Could you check a few things on this model? Use its own coordinates, in mm. Give positions to 0.01 mm unless a question says otherwise; leave off trailing zeros. Order: outer loops, then holes, each group sorted by start corner. A loop starts at its lowest first (then second) coordinate and runs counter-clockwise, first axis right, second up.
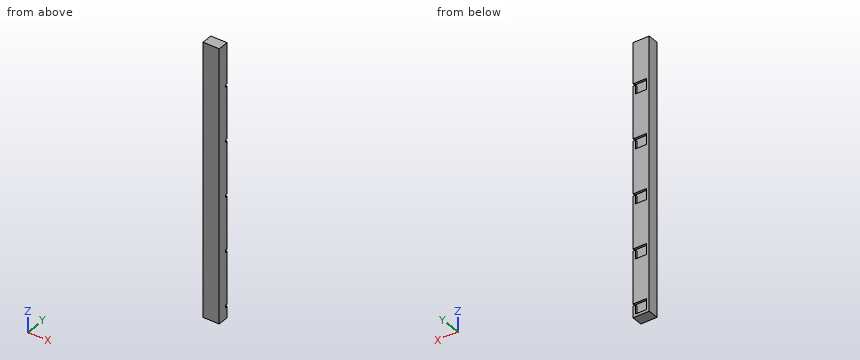
from build123d import *

# Parameters (mm, degrees)
SKETCH1_W           = 15
SKETCH1_H           = 300
BOSS_EXTRUDE1_DEPTH = 10
CUT_EXTRUDE2_DEPTH  = 2
CUT_EXTRUDE3_DEPTH  = 2
CUT_EXTRUDE4_DEPTH  = 2
CUT_EXTRUDE5_DEPTH  = 2
CUT_EXTRUDE6_DEPTH  = 2
SKETCH8_W           = 15
SKETCH8_H           = 10
CUT_EXTRUDE7_DEPTH  = 50


with BuildPart() as part:
    # Sketch1 → Boss-Extrude1 (new body)
    with BuildSketch(Plane(origin=(0, 0, 0), x_dir=(1, 0, 0), z_dir=(0, 1, 0))):
        with Locations((7.5, 150)):
            Rectangle(SKETCH1_W, SKETCH1_H)
    extrude(amount=BOSS_EXTRUDE1_DEPTH)

    # Sketch2 → Cut-Extrude2 (cut)
    with BuildSketch(Plane(origin=(0, 10, 0), x_dir=(1, 0, 0), z_dir=(0, 1, 0))):
        Polygon((2.5, 297.5), (12.5, 297.5), (12.5, 289.5), (15, 289.5), (15, 287.5), (12.5, 287.5), (2.5, 287.5), align=None)
    extrude(amount=-CUT_EXTRUDE2_DEPTH, mode=Mode.SUBTRACT)

    # Sketch3 → Cut-Extrude3 (cut)
    with BuildSketch(Plane(origin=(0, 10, 0), x_dir=(1, 0, 0), z_dir=(0, 1, 0))):
        Polygon((2.5, 247.5), (12.5, 247.5), (12.5, 239.5), (15, 239.5), (15, 237.5), (12.5, 237.5), (2.5, 237.5), align=None)
    extrude(amount=-CUT_EXTRUDE3_DEPTH, mode=Mode.SUBTRACT)

    # Sketch4 → Cut-Extrude4 (cut)
    with BuildSketch(Plane(origin=(0, 10, 0), x_dir=(1, 0, 0), z_dir=(0, 1, 0))):
        Polygon((12.5, 187.5), (15, 187.5), (15, 189.5), (12.5, 189.5), (12.5, 197.5), (2.5, 197.5), (2.5, 187.5), align=None)
    extrude(amount=-CUT_EXTRUDE4_DEPTH, mode=Mode.SUBTRACT)

    # Sketch5 → Cut-Extrude5 (cut)
    with BuildSketch(Plane(origin=(0, 10, 0), x_dir=(1, 0, 0), z_dir=(0, 1, 0))):
        Polygon((12.5, 137.5), (15, 137.5), (15, 139.5), (12.5, 139.5), (12.5, 147.5), (2.5, 147.5), (2.5, 137.5), align=None)
    extrude(amount=-CUT_EXTRUDE5_DEPTH, mode=Mode.SUBTRACT)

    # Sketch6 → Cut-Extrude6 (cut)
    with BuildSketch(Plane(origin=(0, 10, 0), x_dir=(1, 0, 0), z_dir=(0, 1, 0))):
        Polygon((12.5, 87.5), (15, 87.5), (15, 89.5), (12.5, 89.5), (12.5, 97.5), (2.5, 97.5), (2.5, 87.5), align=None)
    extrude(amount=-CUT_EXTRUDE6_DEPTH, mode=Mode.SUBTRACT)

    # Sketch8 → Cut-Extrude7 (cut)
    with BuildSketch(Plane.XY):
        with Locations((7.5, 5)):
            Rectangle(SKETCH8_W, SKETCH8_H)
    extrude(amount=-CUT_EXTRUDE7_DEPTH, mode=Mode.SUBTRACT)


solid = part.part
Item 1: Imagine slicing it at B-B on z = -194. List the corners of the cut face in (x, y) for me, then the cut area to 3 significant figures.
Findings:
outline: (0, 0) - (15, 0) - (15, 10) - (12.5, 10) - (12.5, 8) - (2.5, 8) - (2.5, 10) - (0, 10) - close
area: 130 mm2
Item 2: Please list where this line runs through material, in increasing order: line 1 along Z through (x, y) = (4, 9.25).
Findings:
line 1: z = -300 to -297.5, -287.5 to -247.5, -237.5 to -197.5, -187.5 to -147.5, -137.5 to -97.5, -87.5 to -50
Item 3: For pin 1 (3 mm diameter, centred on y = 8.5, z = -168, fed in from -X); pin 2 (5 mm diameter, centred on x = 6.5, z = -194.5, fed in from +Y), each with a flat end and sliding along its axis, tell me the tip position at first contact or that it passes through.
Findings:
pin 1: stops at x = 0
pin 2: stops at y = 8
Item 4: Imagine slicing it at A-A on x = 10. List the corners of the cut face in (y, z) for me, then the cut area to 3 significant figures.
Findings:
outline: (0, -300) - (10, -300) - (10, -297.5) - (8, -297.5) - (8, -287.5) - (10, -287.5) - (10, -247.5) - (8, -247.5) - (8, -237.5) - (10, -237.5) - (10, -197.5) - (8, -197.5) - (8, -187.5) - (10, -187.5) - (10, -147.5) - (8, -147.5) - (8, -137.5) - (10, -137.5) - (10, -97.5) - (8, -97.5) - (8, -87.5) - (10, -87.5) - (10, -50) - (0, -50) - close
area: 2,400 mm2
